The listing builds one solid part. Answer for the finished solid, in the listing's coordinates (mm). Round coordinates to 2 decimals unless told otherwise and drop trailing zeros. Loops run counter-clockwise (first coordinate to the right, second up) from the corner with the lowest first, then second, coordinate; pieces in that order, holes last. Notation, with made-up numbers: (27.25, -12) -> (55.25, -12) arc R24 cw to (55.25, 5) -> close; hole circle Ø9 at (77.25, 89). An arc over 180 degrees is marked (long way). One line per question, with ' | ' between items.
from build123d import *

# Parameters (mm, degrees)
F0_W     = 400
F0_H     = 90
F0_W_2   = 4
F0_H_2   = 50
F0_R     = 23
F1_DEPTH = 6.35


with BuildPart() as f1:
    # F0 (on Front) → F1 (new body)
    with BuildSketch(Plane.XZ):
        Rectangle(F0_W, F0_H)
        with Locations((-52, 0)):
            Rectangle(F0_W_2, F0_H_2, mode=Mode.SUBTRACT)
        with BuildLine():
            ThreePointArc((31.051097, 11.172706), (32.509123, 5.670705), (33, 0))
            ThreePointArc((33, 0), (32.509123, -5.670705), (31.051097, -11.172706))
            ThreePointArc((31.051097, -11.172706), (33.529177, -13.339893), (34.451838, -16.5))
            ThreePointArc((34.451838, -16.5), (31.285904, -21.711902), (25.201396, -21.304686))
            ThreePointArc((25.201396, -21.304686), (16.5, -28.578838), (5.849702, -32.477392))
            ThreePointArc((5.849702, -32.477392), (5.867172, -32.738436), (5.873, -33))
            ThreePointArc((5.873, -33), (-0.261564, -38.867172), (-5.849702, -32.477392))
            ThreePointArc((-5.849702, -32.477392), (-16.5, -28.578838), (-25.201396, -21.304686))
            ThreePointArc((-25.201396, -21.304686), (-33.665005, -19.4365), (-31.051097, -11.172706))
            ThreePointArc((-31.051097, -11.172706), (-33, 0), (-31.051097, 11.172706))
            ThreePointArc((-31.051097, 11.172706), (-33.665005, 19.4365), (-25.201396, 21.304686))
            ThreePointArc((-25.201396, 21.304686), (-16.5, 28.578838), (-5.849702, 32.477392))
            ThreePointArc((-5.849702, 32.477392), (-0.261564, 38.867172), (5.873, 33))
            ThreePointArc((5.873, 33), (5.867172, 32.738436), (5.849702, 32.477392))
            ThreePointArc((5.849702, 32.477392), (16.5, 28.578838), (25.201396, 21.304686))
            ThreePointArc((25.201396, 21.304686), (31.285904, 21.711902), (34.451838, 16.5))
            ThreePointArc((34.451838, 16.5), (33.529177, 13.339893), (31.051097, 11.172706))
        make_face(mode=Mode.SUBTRACT)
        with Locations((52, 0)):
            Rectangle(F0_W_2, F0_H_2, mode=Mode.SUBTRACT)
        with BuildLine():
            ThreePointArc((31.051097, -11.172706), (32.509123, -5.670705), (33, 0))
            ThreePointArc((33, 0), (32.509123, 5.670705), (31.051097, 11.172706))
            ThreePointArc((31.051097, 11.172706), (23.492671, 13.5635), (25.201396, 21.304686))
            ThreePointArc((25.201396, 21.304686), (16.5, 28.578838), (5.849702, 32.477392))
            ThreePointArc((5.849702, 32.477392), (0, 27.127), (-5.849702, 32.477392))
            ThreePointArc((-5.849702, 32.477392), (-16.5, 28.578838), (-25.201396, 21.304686))
            ThreePointArc((-25.201396, 21.304686), (-23.366936, 19.207066), (-22.705838, 16.5))
            ThreePointArc((-22.705838, 16.5), (-25.418731, 11.549661), (-31.051097, 11.172706))
            ThreePointArc((-31.051097, 11.172706), (-33, 0), (-31.051097, -11.172706))
            ThreePointArc((-31.051097, -11.172706), (-25.418731, -11.549661), (-22.705838, -16.5))
            ThreePointArc((-22.705838, -16.5), (-23.366936, -19.207066), (-25.201396, -21.304686))
            ThreePointArc((-25.201396, -21.304686), (-16.5, -28.578838), (-5.849702, -32.477392))
            ThreePointArc((-5.849702, -32.477392), (0, -27.127), (5.849702, -32.477392))
            ThreePointArc((5.849702, -32.477392), (16.5, -28.578838), (25.201396, -21.304686))
            ThreePointArc((25.201396, -21.304686), (23.492671, -13.5635), (31.051097, -11.172706))
        make_face()
        Circle(F0_R, mode=Mode.SUBTRACT)
    extrude(amount=F1_DEPTH)


solid = f1.part
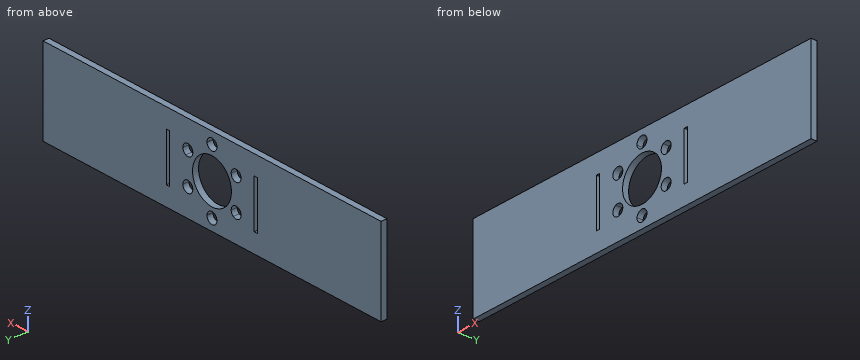
Q1. Find the intervals of material crossed by line 1 (Z direction, x = 0, y = -3.75); line 2 (X direction, y = -3.5, z = -33); line 3 (X direction, y = -0.25, z = -0.5), in increasing order. Write a range as from..to.
Numbers:
line 1: -45..-38.87, -27.13..-23, 23..27.13, 38.87..45 | line 2: -200..-5.87, 5.87..200 | line 3: -200..-54, -50..-22.99, 22.99..50, 54..200
Q2. A cutting plane is placed at C-C on x = -15. Give the vertices of the cut face in (y, z), plus the area to 3 significant figures.
Numbers:
outline: (-6.35, -45) -> (0, -45) -> (0, -17.44) -> (-6.35, -17.44) -> close; (-6.35, 17.44) -> (0, 17.44) -> (0, 45) -> (-6.35, 45) -> close | area: 350 mm^2
Q3. A cutting plane is placed at A-A on z = 0. Give the vertices of the cut face in (x, y).
Numbers:
outline: (-200, -6.35) -> (-54, -6.35) -> (-54, 0) -> (-200, 0) -> close; (-50, -6.35) -> (-23, -6.35) -> (-23, 0) -> (-50, 0) -> close; (23, -6.35) -> (50, -6.35) -> (50, 0) -> (23, 0) -> close; (54, -6.35) -> (200, -6.35) -> (200, 0) -> (54, 0) -> close
Q4. A cutting plane is placed at B-B on y = -3.5. Give the number of separate pieces and of enclosed holes in the cut face, plus the area to 3 significant figures.
Numbers:
separate pieces: 1 | enclosed holes: 9 | area: 33,300 mm^2
